Input: dimensioned drawing with shaded views. Units: mm. Origin: part minimum x, y, z. Give positions to 0.01 mm unless a question says otherwise; leave off trailing zeros. Loops run counter-clockwise (first coordinate to the right, second up) from the corner with the lowest first, then second, coordinate; pieces in that order, holes last.
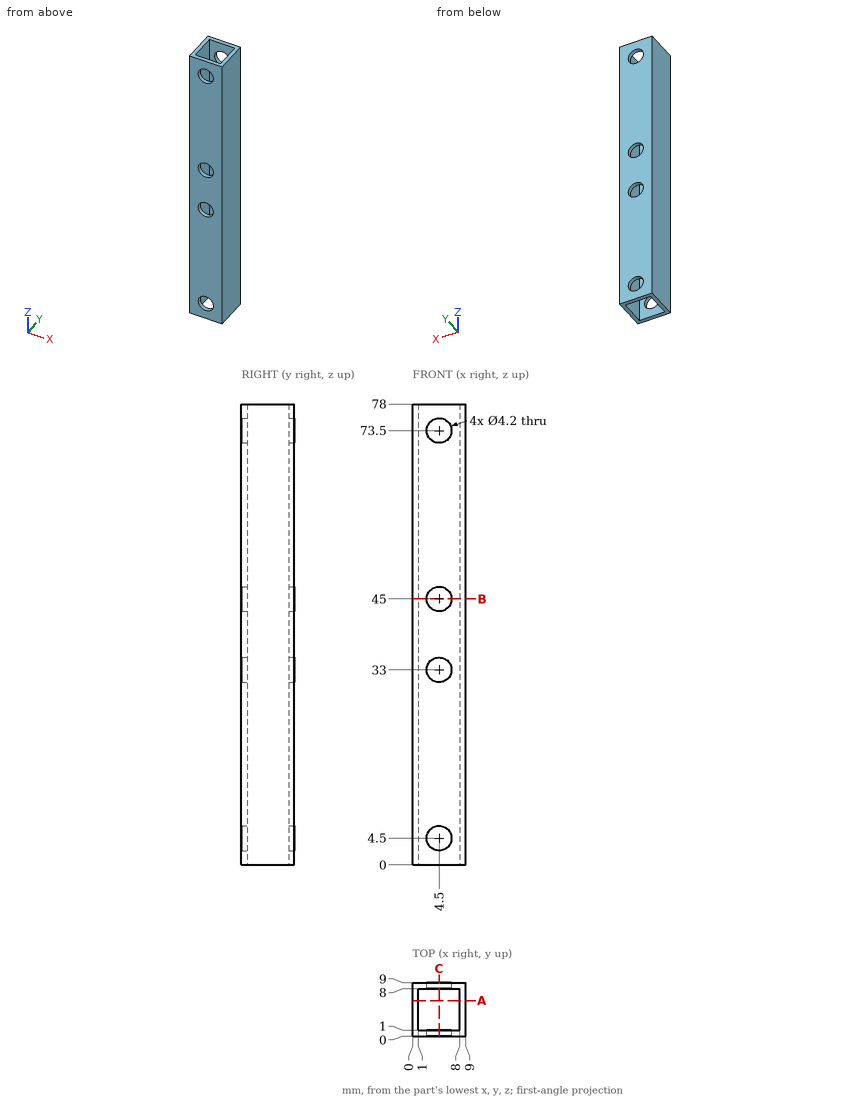
Item 1: Section query C-C on x = 4.5. Give the number of separate pieces and of enclosed holes in the cut face, plus the area to 3 significant figures.
Values follow:
separate pieces: 10
enclosed holes: 0
area: 122 mm2
Item 2: Ray query, probe 1 along Z at (x, y) = (4.5, 8.3); probe 2 along X at (y, z) = (6.25, 70); probe 3 along X at (y, z) = (8.55, 4.5). Return the intervals inside material, ascending.
Values follow:
probe 1: z = 0 to 2.4, 6.6 to 30.9, 35.1 to 42.9, 47.1 to 71.4, 75.6 to 78
probe 2: x = 0 to 1, 8 to 9
probe 3: x = 0 to 2.4, 6.6 to 9
Item 3: Section query A-A on y = 6. Return loops of the section in (x, z).
Values follow:
outline: (0, 0) - (1, 0) - (1, 78) - (0, 78) - close; (8, 0) - (9, 0) - (9, 78) - (8, 78) - close
Item 4: Section query B-B on z = 45. Return loops of the section in (x, y), plus the area to 3 significant figures.
Values follow:
outline: (0, 0) - (2.4, 0) - (2.4, 1) - (1, 1) - (1, 8) - (2.4, 8) - (2.4, 9) - (0, 9) - close; (6.6, 0) - (9, 0) - (9, 9) - (6.6, 9) - (6.6, 8) - (8, 8) - (8, 1) - (6.6, 1) - close
area: 23.6 mm2
